```python
from build123d import *

# Parameters (mm, degrees)
RECTANGLE001_W   = 27
RECTANGLE001_H   = 12
EXTRUDE002_DEPTH = 1
CIRCLE_R         = 2.5
EXTRUDE001_DEPTH = 10
RECTANGLE_W      = 30
RECTANGLE_H      = 15
EXTRUDE_DEPTH    = 4


with BuildPart() as extrude002:
    # Rectangle001 → Extrude002 (new body)
    with BuildSketch(Plane(origin=(-1.345388, -1.581388, 4), x_dir=(1, 0, 0), z_dir=(0, 0, 1))):
        with Locations((13.5, 6)):
            Rectangle(RECTANGLE001_W, RECTANGLE001_H)
    extrude(amount=-EXTRUDE002_DEPTH)


with BuildPart() as cone:
    # Cone → Cone (revolve)
    with BuildSketch(Plane(origin=(6.926492, 4.418612, 0), x_dir=(1, 0, 0), z_dir=(0, -1, 0))):
        Polygon((0, 0), (2.5, 0), (5, 3), (0, 3), align=None)
    revolve(axis=Axis((6.926492, 4.418612, 0), (0, 0, 1)))


with BuildPart() as extrude001:
    # Circle → Extrude001 (new body)
    with BuildSketch(Plane(origin=(6.926492, 4.418612, 0), x_dir=(1, 0, 0), z_dir=(0, 0, 1))):
        Circle(CIRCLE_R)
    extrude(amount=EXTRUDE001_DEPTH)


with BuildPart() as cut002:
    # Rectangle → Extrude (new body)
    with BuildSketch(Plane(origin=(-3.073508, -3.081388, 0), x_dir=(1, 0, 0), z_dir=(0, 0, 1))):
        with Locations((15, 7.5)):
            Rectangle(RECTANGLE_W, RECTANGLE_H)
    extrude(amount=EXTRUDE_DEPTH)

    # Cut: cut Extrude001
    add(extrude001.part, mode=Mode.SUBTRACT)

    # Cut001: cut Cone
    add(cone.part, mode=Mode.SUBTRACT)

    # Cut002: cut Extrude002
    add(extrude002.part, mode=Mode.SUBTRACT)


solid = cut002.part
```
Model file for the job. Use its own axes, mm. A direction names the side the tool comes from. Give positions to 0.01 mm unless a question says otherwise; leave off trailing zeros. Loops run counter-clockwise (first coordinate to the right, second up) from the corner with the lowest first, then second, coordinate; pieces in that order, holes last. Notation, with made-up numbers: (16.5, 36) - (27.5, 36) arc R19 cw to (27.5, 50) - close; hole circle Ø10 at (81, -13.75). An arc over 180 degrees is marked (long way). One line per item, written item: value. Start each with the question number.
1. Slice it at C-C (x = 15). List the corners of the cut face in (y, z).
2. Pull direction Y, two halves, no side cores. Call faces 3 (the flat face through (12, 11.919, 2)), 4 (the conical face through (9.38, 3.4, 0.19)), 5 (the flat face through (10, -2, 4)): pulls with the +Y half, pulls with the -Y half, needs draft (parallel to the pull), parting line crosses it, or undercut.
3. Pin check, flat tip, straight feed: pin 1 (3.5 mm diameter, centred on x = 17, y = 2, fed in from +Z). Stop position of the tip, or through.
4. Which spindle directions (+Z, -Z, +X, -X, +Y, -Y) get a long thin tool onto all of the face, cutting with end or side? Do faces 1 (the flat face through (15, 5, 3)), 2 (the flat face through (26.926, 4, 2)). Say none if no direction does.
5. Probe L1, parallel to X at y = -1.25, z = 3.7; L2, parallel to Y at x = 25, z = 3.35; L3, parallel to Z at x = 0, y = 8.75. List the from-to ranges inside material, lowest first. Write a range as from..to.
6. Slice it at B-B (z = 1.8). List the corners of the cut face in (x, y).
7. Slice it at D-D (z = 0.4). List the corners of the cut face in (x, y).
8. Slice it at A-A (y = -1). List the corners of the cut face in (x, z).
Solution:
1. outline: (-3.08, 0) - (11.92, 0) - (11.92, 4) - (10.42, 4) - (10.42, 3) - (-1.58, 3) - (-1.58, 4) - (-3.08, 4) - close
2. face 3: pulls with the +Y half
2. face 4: undercut
2. face 5: needs draft
3. pin 1: stops at z = 3
4. face 1: +Z
4. face 2: +Z, -Z, +X, +Y, -Y
5. L1: x = -3.07..-1.35, 25.65..26.93
5. L2: y = -3.08..-1.58, 10.42..11.92
5. L3: z = 0..3
6. outline: (-3.07, -3.08) - (26.93, -3.08) - (26.93, 11.92) - (-3.07, 11.92) - close; hole circle Ø8 at (6.93, 4.42)
7. outline: (-3.07, -3.08) - (26.93, -3.08) - (26.93, 11.92) - (-3.07, 11.92) - close; hole circle Ø5.67 at (6.93, 4.42)
8. outline: (-3.07, 0) - (26.93, 0) - (26.93, 4) - (25.65, 4) - (25.65, 3) - (-1.35, 3) - (-1.35, 4) - (-3.07, 4) - close
